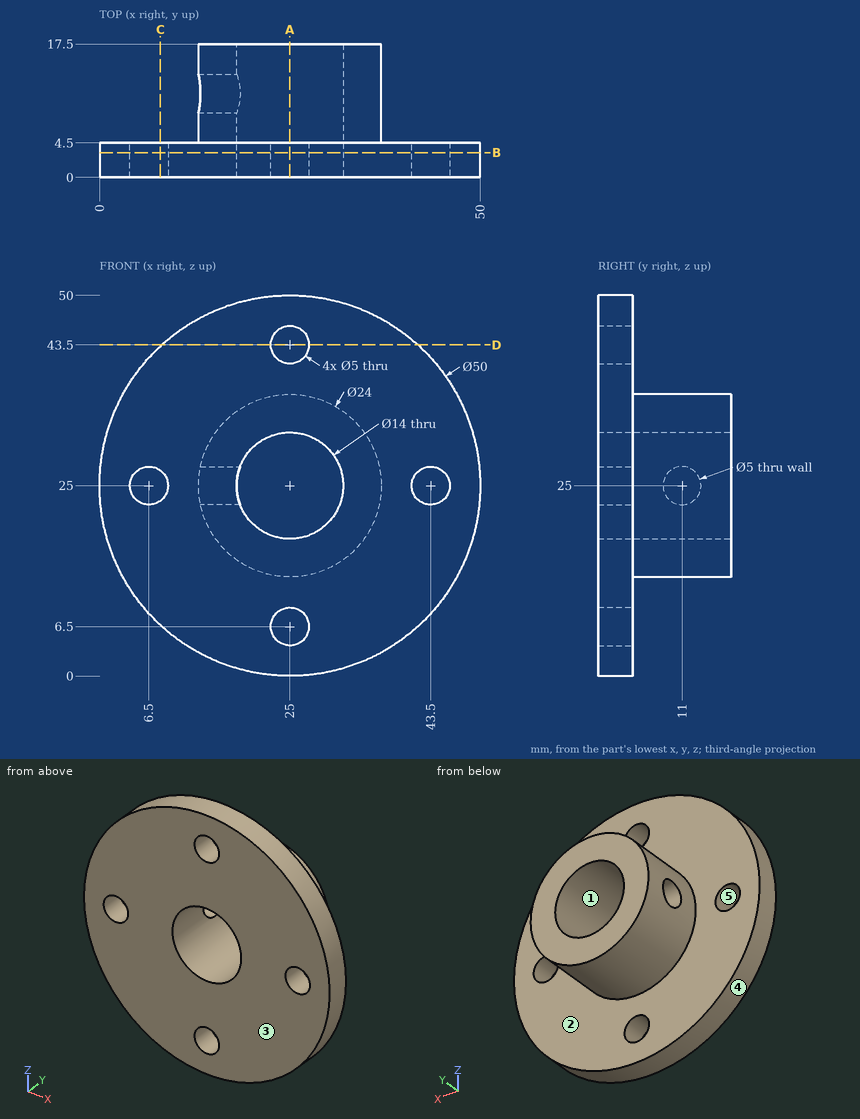
Job drawing, mm, ordinate dimensions from the low corner. One solid piece. A direction names the side the tool comes from. Give positions to 0.01 mm unless a question says otherwise; leave off trailing zeros. Order: outer loops, then holes, each group sorted by start corner. A loop starts at its lowest first (then second) coordinate and runs counter-clockwise, first axis right, second up. Notation, with made-up numbers: (14.25, 49) - (20.25, 49) arc R12 ccw to (20.25, 68) - close; hole circle Ø8 at (3.5, -38). An arc over 180 degrees is marked (long way). Answer in a Markdown table with one row per item.
1. Pull direction X, two halves, no side cores. Call the marked faces 3, 4 and 5: pulls with the +X half, pulls with the -X half, needs draft (parallel to the pull), parting line crosses it, or undercut.
Data:
| item | result |
|---|---|
| face 3 | needs draft |
| face 4 | parting line crosses it |
| face 5 | undercut |
2. Probe probe 1 along X at (y, z) = (3.35, 25); probe 2 along X at (y, z) = (5.5, 25); probe 3 along Y at (x, z) = (37.5, 21.5). List the from-to ranges inside material, lowest first. Write a range as [from, to].
Data:
| item | result |
|---|---|
| probe 1 | x = [0, 4], [9, 18], [32, 41], [46, 50] |
| probe 2 | x = [13, 18], [32, 37] |
| probe 3 | y = [0, 4.5] |
3. Saw through at D-D, the plane z = 43.5. Give the cut face in (x, y), plus the area to 3 significant figures.
Data:
| item | result |
|---|---|
| outline | (8.18, 0) - (22.5, 0) - (22.5, 4.5) - (8.18, 4.5) - close; (27.5, 0) - (41.82, 0) - (41.82, 4.5) - (27.5, 4.5) - close |
| area | 129 mm² |
4. Flat gauge pins, fed straight in: pin 1 (5 mm diameter, centred on x = 34, y = 3.5, fed in from +Z); pin 2 (6 mm diameter, centred on x = 25, z = 6.5, fed in from +Y); pin 3 (4 mm diameter, centred on y = 4, z = 34.5, fed in from +X). Where does each tip first touch, or does it go through?
Data:
| item | result |
|---|---|
| pin 1 | stops at z = 49.14 |
| pin 2 | stops at y = 4.5 |
| pin 3 | stops at x = 48.85 |
5. Saw through at B-B, the plane y = 3.25. Give the cut face in (x, z).
Data:
| item | result |
|---|---|
| outline | circle Ø50 at (25, 25); hole circle Ø5 at (6.5, 25); hole circle Ø14 at (25, 25); hole circle Ø5 at (25, 6.5); hole circle Ø5 at (25, 43.5); hole circle Ø5 at (43.5, 25) |
6. Saw through at C-C, the plane x = 8. Give the cut face in (y, z).
Data:
| item | result |
|---|---|
| outline | (0, 6.67) - (4.5, 6.67) - (4.5, 23) - (0, 23) - close; (0, 27) - (4.5, 27) - (4.5, 43.33) - (0, 43.33) - close |
7. Saw through at A-A, the plane x = 25. Give the cut face in (y, z).
Data:
| item | result |
|---|---|
| outline | (0, 0) - (4.5, 0) - (4.5, 4) - (0, 4) - close; (0, 9) - (4.5, 9) - (4.5, 13) - (17.5, 13) - (17.5, 18) - (0, 18) - close; (0, 32) - (17.5, 32) - (17.5, 37) - (4.5, 37) - (4.5, 41) - (0, 41) - close; (0, 46) - (4.5, 46) - (4.5, 50) - (0, 50) - close |
8. Tool access for the marked faces 1 and 2: list every direction of +Z, -Z, +X, -X, +Y, -Y with a clear straight run to the whole face (end or side of a thin tool).
Data:
| item | result |
|---|---|
| face 1 | +Y, -Y |
| face 2 | +Y |
